The listing builds one solid part. Answer for the finished solid, in the listing's coordinates (mm). A direction names the side the tool comes from. Give positions to 0.01 mm unless a question says otherwise; leave off trailing zeros. Loops run counter-clockwise (first coordinate to the right, second up) from the corner with the lowest first, then second, coordinate; pieces in that order, holes last.
Item 1: Consider line 1 along X through (y, z) = (8, 1); line 2 along X through (y, z) = (7, 0); line 3 along Y through (x, z) = (-2.75, -3.25). Determine where each line is inside the solid, lowest interval first.
Item 2: Section A-A, the plane y = 7 is taken. Give the vertices of the cut face in (x, z), and give its area (3 significant figures).
Item 3: The mould has two halves that part along X. Classify faces 4 (the face through (-1.08, -1.51, 0.63)), 5 (the face through (0, -0.8, 4)), 6 (the face through (0, 8, 2)): pulls with the +X half, pulls with the -X half, needs draft (parallel to the pull), parting line crosses it, or undercut.
Item 4: Each of these flat-tipped pins is pushed along its axis until it touches: pin 1 Ø1.5 at (x, y) = (3, 7) entering from +Z; pin 2 Ø5 at (x, y) = (-3, 13) entering from -Z; pin 3 Ø3 at (x, z) = (-2, -3.5) entering from +Y. Where does it stop, or does it pass through?
Item 5: A tool of negligible diameter and unlimited length cuts with its end or side. For faces 1 (the face through (1.08, -1.51, -0.63)), 2 (the face through (0, 16, 0)), 3 (the face through (2, 0, 2)), from which of +Z, -Z, +X, -X, +Y, -Y can it reach the whole face along a straight path? Write none if from no direction.
Solid Edge part; units mm, degrees
sketch "Sketch1" plane through (0, 0, 0) normal (0, 0, 1) x (1, 0, 0)
  line L0 (2, 0) -> (2, 16)
  line L1 (0, 16) -> (2, 16)
  line L2 (0, 0) -> (0, 16)
  line L3 (0, 0) -> (0, -2.2)
  line L4 (0, -2.2) -> (3.6, -2.2)
  line L5 (3.6, -2.2) -> (3.6, 0)
  line L6 (3.6, 0) -> (2, 0)
revolve "RevolvedProtrusion1" add sketch "Sketch1" angle 360 about axis through (0, 0, 0) along (0, 1, 0)
sketch "Sketch2" plane through (0, 0, 0) normal (1, 0, 0) x (0, 1, 0)
  line L0 (-2.2, 1.9365) -> (-0.9, 1.9365)
  line L1 (0.218, 0) -> (-0.9, 1.9365)
  line L2 (-2.2, 0) -> (0.218, 0)
  line L3 (-2.2, 0) -> (-2.2, 1.9365)
revolve "RevolvedCutout1" cut sketch "Sketch2" angle 360 about axis through (0, -4.5, 0) along (0, 1, 0)
sketch "Sketch3" plane through (0, -2.2, 0) normal (0, -1, 0) x (0, 0, 1)
  circle A0 centre (0, 0) radius 1.9365
  line L0 (-1.25, -0.7217) -> (0, -1.4434)
  line L1 (0, -1.4434) -> (1.25, -0.7217)
  line L2 (1.25, -0.7217) -> (1.25, 0.7217)
  line L3 (1.25, 0.7217) -> (0, 1.4434)
  line L4 (0, 1.4434) -> (-1.25, 0.7217)
  line L5 (-1.25, 0.7217) -> (-1.25, -0.7217)
extrude "Protrusion1" add sketch "Sketch3" against normal up to next
sketch "Sketch4" plane through (0, 0, 0) normal (0, 0, 1) x (1, 0, 0)
  line L0 (-1.4434, -2.2) -> (0, -2.2)
  line L1 (0, -2.2) -> (0, -1.8132)
  line L2 (0, -1.8132) -> (-1.4434, -2.2)
revolve "RevolvedCutout2" cut sketch "Sketch4" angle 360 about axis through (0, -4.5, 0) along (0, 1, 0)
fillet "Round1" radius 0.2 1 edges at (0, 0, -2)
chamfer "倒斜角_2" distance 0.2667 angle 45 1 edges at (0, 16, -2)
cosmetic_thread "螺纹_3" thread depth 15.5333
sketch "Sketch5" plane through (0, 0, 0) normal (0, 0, 1) x (1, 0, 0)
  arc A0 (-1.9153, -2.2) -> (-3.6, 0) centre (-1.3212, 0) cw
revolve "RevolvedCutout3" cut sketch "Sketch5" angle 360 about axis through (0, 0, 0) along (0, -1, 0) material side at (-3.1701, -1.4159, 0)
sketch "Sketch6" plane through (0, 0, 0) normal (0, 0, 1) x (1, 0, 0)
  arc A0 (-4.3, 0) -> (-4.3, -0.8) centre (-4.3, -0.4) ccw
  line L0 (-4.3, -0.8) -> (0, -0.8)
  line L1 (0, -0.8) -> (0, 0)
  line L2 (0, 0) -> (-4.3, 0)
revolve "RevolvedProtrusion2" add sketch "Sketch6" angle 360 about axis through (0, -0.7, 0) along (0, 1, 0)
properties part number "N2611-0316" material "铝 1060"
Worked answers:
1. line 1: x = -1.73 to 1.73
1. line 2: x = -2 to 2
1. line 3: y = -0.8 to 0
2. outline: circle Ø4 at (0, 0)
2. area: 12.6 mm2
3. face 4: undercut
3. face 5: needs draft
3. face 6: parting line crosses it
4. pin 1: passes through
4. pin 2: stops at z = -1.94
4. pin 3: stops at y = 0
5. face 1: -Y
5. face 2: +Z, -Z, +X, -X, +Y
5. face 3: +Y
